Geometry: final body of the model. Coordinates: model frame, mm. A direction names the side the tool comes from. Round coordinates to 2 decimals unless told otherwise and drop trailing zeros. Write each loop counter-clockwise with the first axis right and the second up, starting at its lowest first coordinate (ties: lowest second). Pieces come first, ordered by that corner, then holes. Notation, with made-up numbers: (10.5, 25.5) - (44.5, 25.5) arc R29 cw to (44.5, 48.5) - close; hole circle Ø4 at (51, -10). An arc over 180 degrees is marked (long way). Write each question's results on one line, items separated by ' | '.
from build123d import *

# Parameters (mm, degrees)
F1_DEPTH = 381
F2_R     = 6.35
F3_DEPTH = 127.001
F4_W     = 50.8
F4_H     = 254
F5_DEPTH = 127.001
F7_DEPTH = 63.5


with BuildPart() as f1:
    # F0 (on Front) → F1 (new body)
    with BuildSketch(Plane.XZ):
        Polygon((190.5, -228.6), (190.5, 228.6), (139.7, 228.6), (139.7, 25.4), (-63.5, 25.4), (-63.5, -101.6), (-190.5, -101.6), (-190.5, -228.6), align=None)
    extrude(amount=F1_DEPTH)

    # F2 (on face) → F3 (cut, through all)
    with BuildSketch(Plane.XY.offset(-101.6)):
        with Locations((-139.7, -190.5)):
            Circle(F2_R)
    extrude(amount=-F3_DEPTH, mode=Mode.SUBTRACT)

    # F4 (on face) → F5 (cut, through all)
    with BuildSketch(Plane.XY.offset(-101.6)):
        with Locations((-101.6, -190.5)):
            Rectangle(F4_W, F4_H)
    extrude(amount=-F5_DEPTH, mode=Mode.SUBTRACT)

    # F6 (on face) → F7 (cut)
    with BuildSketch(Plane(origin=(139.7, 0, 0), x_dir=(0, -1, 0), z_dir=(-1, 0, 0))):
        with BuildLine():
            Line((88.9, 139.7), (292.1, 139.7))
            ThreePointArc((292.1, 139.7), (317.5, 165.1), (292.1, 190.5))
            Line((292.1, 190.5), (88.9, 190.5))
            ThreePointArc((88.9, 190.5), (63.5, 165.1), (88.9, 139.7))
        make_face()
    extrude(amount=-F7_DEPTH, mode=Mode.SUBTRACT)


solid = f1.part
Q1. Access query for faces 1 (the flat face through (165, -189, 139.7)), 2 (the flat face through (40, -188, 25.4)), 3 (the flat face through (-3, -188, -228.6)), 4 (the flat face through (-127, -192, -164)). Directions: +Z, -Z, +X, -X, +Y, -Y. A direction counts if a zero-diameter tool reaches every point of the face in a straight line with its end or side. Return the directions, or none.
Answer block:
face 1: +X, -X | face 2: +Z, -X, +Y, -Y | face 3: -Z, +X, -X, +Y, -Y | face 4: +Z, -Z
Q2. Pin query (flat end, axial travel): pin 1 (4 mm diameter, centred on x = -71, y = -223.5, fed in from +Z); pin 2 (8 mm diameter, centred on x = -139, z = -101.5, fed in from +Y); pin 3 (5 mm diameter, centred on y = -298, z = 11.5, fed in from -X). Return the tip coordinate at first contact, or that it passes through.
Answer block:
pin 1: z = -101.6 | pin 2: y = 0 | pin 3: x = -63.5
Q3. Section query B-B, the plane z = 165.1. Return loops of the section in (x, y).
Answer block:
outline: (139.7, -381) - (190.5, -381) - (190.5, -317.5) - (139.7, -317.5) - close; (139.7, -63.5) - (190.5, -63.5) - (190.5, 0) - (139.7, 0) - close
Q4. Mould query, pull axis Y, two halves, no side actions, for faces 5 (the flat face through (-102, -317.5, -164)), 6 (the flat face through (40, 0, -98)), 7 (the flat face through (139.7, -188, 128)). Classes: pulls with the +Y half, pulls with the -Y half, needs draft (parallel to the pull), parting line crosses it, or undercut.
Answer block:
face 5: undercut | face 6: pulls with the +Y half | face 7: needs draft
Q5. Section query A-A, the plane x = -139.7. Return loops of the section in (y, z), plus the area to 3 significant figures.
Answer block:
outline: (-381, -228.6) - (-196.85, -228.6) - (-196.85, -101.6) - (-381, -101.6) - close; (-184.15, -228.6) - (0, -228.6) - (0, -101.6) - (-184.15, -101.6) - close | area: 46,800 mm2
Q6. Section query D-D, the plane z = -162. Return loops of the section in (x, y), plus the area to 3 significant figures.
Answer block:
outline: (-190.5, -381) - (190.5, -381) - (190.5, 0) - (-190.5, 0) - close; hole circle Ø12.7 at (-139.7, -190.5); hole (-127, -317.5) - (-76.2, -317.5) - (-76.2, -63.5) - (-127, -63.5) - close | area: 132,000 mm2
Q7. Ray query, line 1 along X through (y, z) = (-190, -182); line 2 along Y through (x, z) = (-139.7, -154); line 3 along Z through (x, y) = (159, -119). Return the intervals inside material, ascending.
Answer block:
line 1: -190.5 to -146.03, -133.37 to -127, -76.2 to 190.5 | line 2: -381 to -196.85, -184.15 to 0 | line 3: -228.6 to 139.7, 190.5 to 228.6
Q8. Section query C-C, the plane y = -190.5. Return loops of the section in (x, z), plus the area to 3 significant figures.
Answer block:
outline: (-190.5, -228.6) - (-146.05, -228.6) - (-146.05, -101.6) - (-190.5, -101.6) - close; (-133.35, -228.6) - (-127, -228.6) - (-127, -101.6) - (-133.35, -101.6) - close; (-76.2, -228.6) - (190.5, -228.6) - (190.5, 139.7) - (139.7, 139.7) - (139.7, 25.4) - (-63.5, 25.4) - (-63.5, -101.6) - (-76.2, -101.6) - close; (139.7, 190.5) - (190.5, 190.5) - (190.5, 228.6) - (139.7, 228.6) - close | area: 80,300 mm2
